from build123d import *

# Parameters (mm, degrees)
SKETCH014_W     = 83
SKETCH014_H     = 33.5
PAD008_DEPTH    = 29
CHAMFER001_SIZE = 10
SKETCH018_R     = 18.052065
POCKET006_DEPTH = 33.501


with BuildPart() as part:
    # Sketch014 → Pad008 (new body, symmetric)
    with BuildSketch(Plane.YZ):
        with Locations((-41.5, 0)):
            Rectangle(SKETCH014_W, SKETCH014_H)
    extrude(amount=PAD008_DEPTH, both=True)

    # Chamfer001
    chamfer001_edges = [part.edges().sort_by_distance(p)[0] for p in [
        (-29, -83, 0),
        (29, -83, 0),
    ]]
    chamfer(chamfer001_edges, length=CHAMFER001_SIZE)

    # Sketch018 (on Face8 of Chamfer001) → Pocket006 (cut, through all)
    with BuildSketch(Plane(origin=(0, 0, 16.75), x_dir=(0, -1, 0), z_dir=(0, 0, 1))):
        with Locations((59.696613, 0)):
            Circle(SKETCH018_R)
    extrude(amount=-POCKET006_DEPTH, mode=Mode.SUBTRACT)


solid = part.part
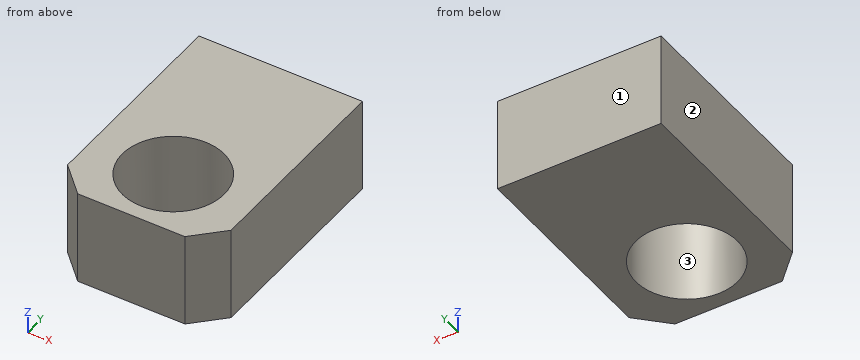
Could you check a few things on this model? Use its own coordinates, in mm. Face numbers are marked on the shaded views. Give positions to 0.01 mm unless a question says otherwise; leave off trailing zeros. Order: outer loops, then holes, each group sorted by start corner. A loop starts at its lowest first (then second) coordinate and runs counter-clockwise, first axis right, second up.
1. Suppose I cut it at A-A (x = 0). List the corners of the cut face in (y, z) for me, plus the area to 3 significant figures.
2. I need wall thicknesses on L1, parallel to Y at x = -2.5, z = 9; L2, parallel to Y at x = -3, z = 13; L3, parallel to X at y = -69.5, z = 0. Which ranges of each line are inside material? Lowest first, please.
3. Suppose I cut it at C-C (x = -11.5). List the corners of the cut face in (y, z) for me.
4. We'd pull the mould along Y, two halves only. Please class the marked faces 1, 2 and 3: pulls with the +Y half, pulls with the -Y half, needs draft (parallel to the pull), parting line crosses it, or undercut.
5. Suppose I cut it at B-B (z = -13). List the corners of the cut face in (x, y) for me, plus the area to 3 significant figures.
Solved:
1. outline: (-83, -16.75) - (-77.75, -16.75) - (-77.75, 16.75) - (-83, 16.75) - close; (-41.64, -16.75) - (0, -16.75) - (0, 16.75) - (-41.64, 16.75) - close
1. area: 1,570 mm2
2. L1: y = -83 to -77.57, -41.82 to 0
2. L2: y = -83 to -77.5, -41.9 to 0
2. L3: x = -29 to -15.16, 15.16 to 29
3. outline: (-83, -16.75) - (-73.61, -16.75) - (-73.61, 16.75) - (-83, 16.75) - close; (-45.78, -16.75) - (0, -16.75) - (0, 16.75) - (-45.78, 16.75) - close
4. face 1: pulls with the +Y half
4. face 2: needs draft
4. face 3: undercut
5. outline: (-29, -73) - (-19, -83) - (19, -83) - (29, -73) - (29, 0) - (-29, 0) - close; hole circle Ø36.1 at (0, -59.7)
5. area: 3,690 mm2
